The listing builds one solid part. Answer for the finished solid, in the listing's coordinates (mm). A direction names the side the tool comes from. Coordinates: 2 decimals unless noted, no trailing zeros.
from build123d import *

# Parameters (mm, degrees)
ESQUISSE2_R             = 1.25
BOSS_EXTRU_1_DEPTH      = 125
ENL_V_MAT_EXTRU_1_DEPTH = 11


with BuildPart() as part:
    # Esquisse2 → Boss.-Extru.1 (new body)
    with BuildSketch(Plane.XY):
        Polygon((-1, -2), (1, -2), (3.383507185, -4), (1.5, -4), (1.5, -5), (5, -5), (5, -1.5), (4, -1.5), (4, -3.383507185), (2, -1), (2, 1), (4, 3.383507185), (4, 1.5), (5, 1.5), (5, 5), (1.5, 5), (1.5, 4), (3.383507185, 4), (1, 2), (-1, 2), (-3.383507185, 4), (-1.5, 4), (-1.5, 5), (-5, 5), (-5, 1.5), (-4, 1.5), (-4, 3.383507185), (-2, 1), (-2, -1), (-4, -3.383507185), (-4, -1.5), (-5, -1.5), (-5, -5), (-1.5, -5), (-1.5, -4), (-3.383507185, -4), align=None)
        Circle(ESQUISSE2_R, mode=Mode.SUBTRACT)
    extrude(amount=BOSS_EXTRU_1_DEPTH)

    # Esquisse3 → Enlèv. mat.-Extru.1 (cut, through all)
    with BuildSketch(Plane(origin=(0, 5, 0), x_dir=(1, 0, 0), z_dir=(0, 1, 0))):
        Polygon((-5, 0), (5, 0), (5, -4.142135624), align=None)
        Polygon((5, -120.857864376), (-5, -125), (5, -125), align=None)
    extrude(amount=-ENL_V_MAT_EXTRU_1_DEPTH, mode=Mode.SUBTRACT)


solid = part.part
(1) The mould has two halves that part along X. Classify faces 4 (the flat face through (-2, 0, 62)), 5 (the flat face through (2.208, 3.014, 61.66)), 6 (the flat face through (5, -3, 62)): pulls with the +X half, pulls with the -X half, needs draft (parallel to the pull), parting line crosses it, or undercut.
(2) Find the intervals of material crossed by probe 1 along X at (y, z) = (0, 69); probe 2 along X at (y, z) = (-4.25, 57), in increasing order.
(3) A tool of negligible diameter and unlimited length cuts with its end or side. For faces 1 (the flat face through (0, -2, 62)), 2 (the flat face through (2, 0, 62)), 3 (the flat face through (0, 2, 62)), from which of +Z, -Z, +X, -X, +Y, -Y can it reach the whole face along a straight path? Write none if from no direction.
(4) Given pin 1 Ø1 at (y, z) = (0, 67.5) entering from +X; pin 2 Ø1.5 at (x, y) = (0, 0) entering from -Z, each flat-ended and moving along its own axis, determine where each tip first touches the part or whether it passes through.
Resolved:
1. face 4: pulls with the -X half
1. face 5: undercut
1. face 6: pulls with the +X half
2. probe 1: x = -2 to -1.25, 1.25 to 2
2. probe 2: x = -5 to -1.5, 1.5 to 5
3. face 1: +Z, -Z, -Y
3. face 2: +Z, -Z, +X
3. face 3: +Z, -Z, +Y
4. pin 1: stops at x = 2
4. pin 2: passes through
